Can you work these out from the drawing? Everything is in mm from the part's minimum corner. Coordinates: 2 decimals unless noted, no trailing zeros. Order: outer loops, then holes, each group sorted by start corner. A loop starts at its lowest first (then second) coordinate and runs counter-clockwise, first axis right, second up. Notation, with made-up numbers: (88, -33) - (99, -33) arc R19 ccw to (99, -25) - close; hole circle Ø6 at (17, 23). An arc over 180 degrees is marked (long way). Answer as CSV lines item,"result". Start each with the question number.
Q1. Suppose I cut it at B-B (z = 0.4). Please give me the cut outline in (x, y), then the cut area to 3 significant figures.
Q2. I need wall thicknesses on line 1 (Y direction, x = 2.5, z = 1.25); line 2 (Y direction, x = 2.25, z = 0.3); line 3 (X direction, y = 1.5, z = 1.55). Which ranges of each line are inside material? Lowest first, please.
Q3. Suppose I cut it at A-A (y = 23.5). Please give me the cut outline in (x, z), then the cut area to 3 significant figures.
Q4. Suppose I cut it at C-C (x = 2.5). Please give me the cut outline in (y, z).
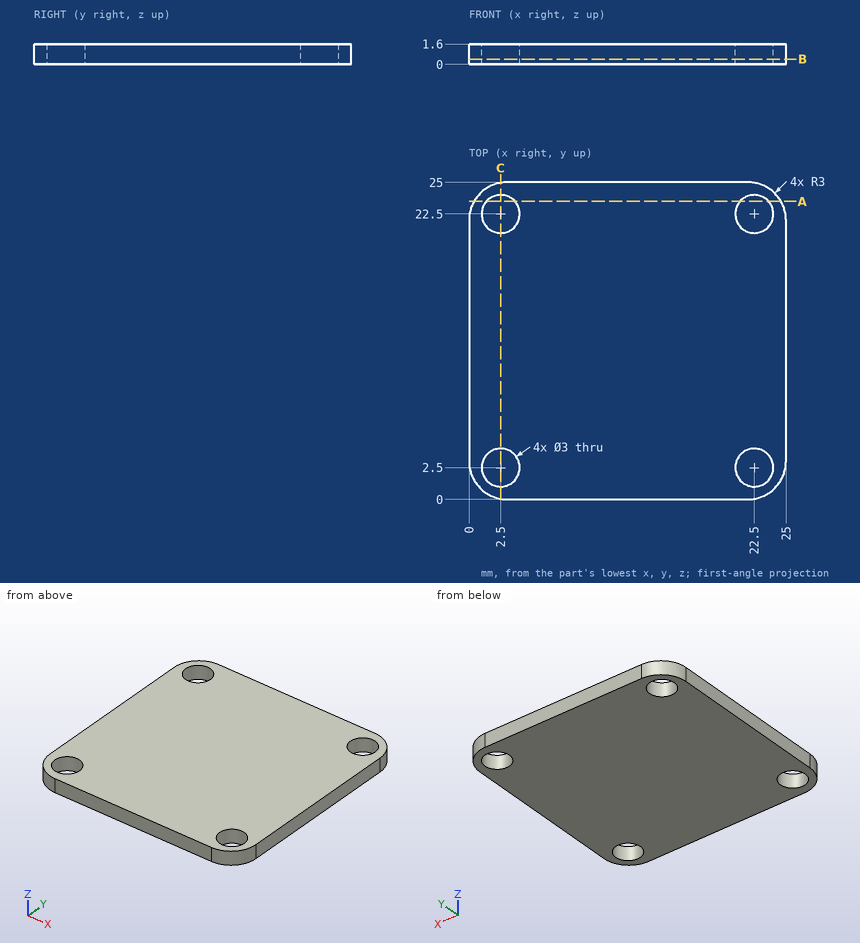
Here are the results:
1,outline,"(0, 3) arc R3 ccw to (3, 0) - (22, 0) arc R3 ccw to (25, 3) - (25, 22) arc R3 ccw to (22, 25) - (3, 25) arc R3 ccw to (0, 22) - close; hole circle Ø3 at (2.5, 2.5); hole circle Ø3 at (2.5, 22.5); hole circle Ø3 at (22.5, 2.5); hole circle Ø3 at (22.5, 22.5)"
1,area,"589 mm²"
2,line 1,"y = 0.04 to 1, 4 to 21, 24 to 24.96"
2,line 2,"y = 0.1 to 1.02, 3.98 to 21.02, 23.98 to 24.9"
2,line 3,"x = 0.4 to 1.38, 3.62 to 21.38, 23.62 to 24.6"
3,outline,"(0.4, 0) - (1.38, 0) - (1.38, 1.6) - (0.4, 1.6) - close; (3.62, 0) - (21.38, 0) - (21.38, 1.6) - (3.62, 1.6) - close; (23.62, 0) - (24.6, 0) - (24.6, 1.6) - (23.62, 1.6) - close"
3,area,"31.6 mm²"
4,outline,"(0.04, 0) - (1, 0) - (1, 1.6) - (0.04, 1.6) - close; (4, 0) - (21, 0) - (21, 1.6) - (4, 1.6) - close; (24, 0) - (24.96, 0) - (24.96, 1.6) - (24, 1.6) - close"
